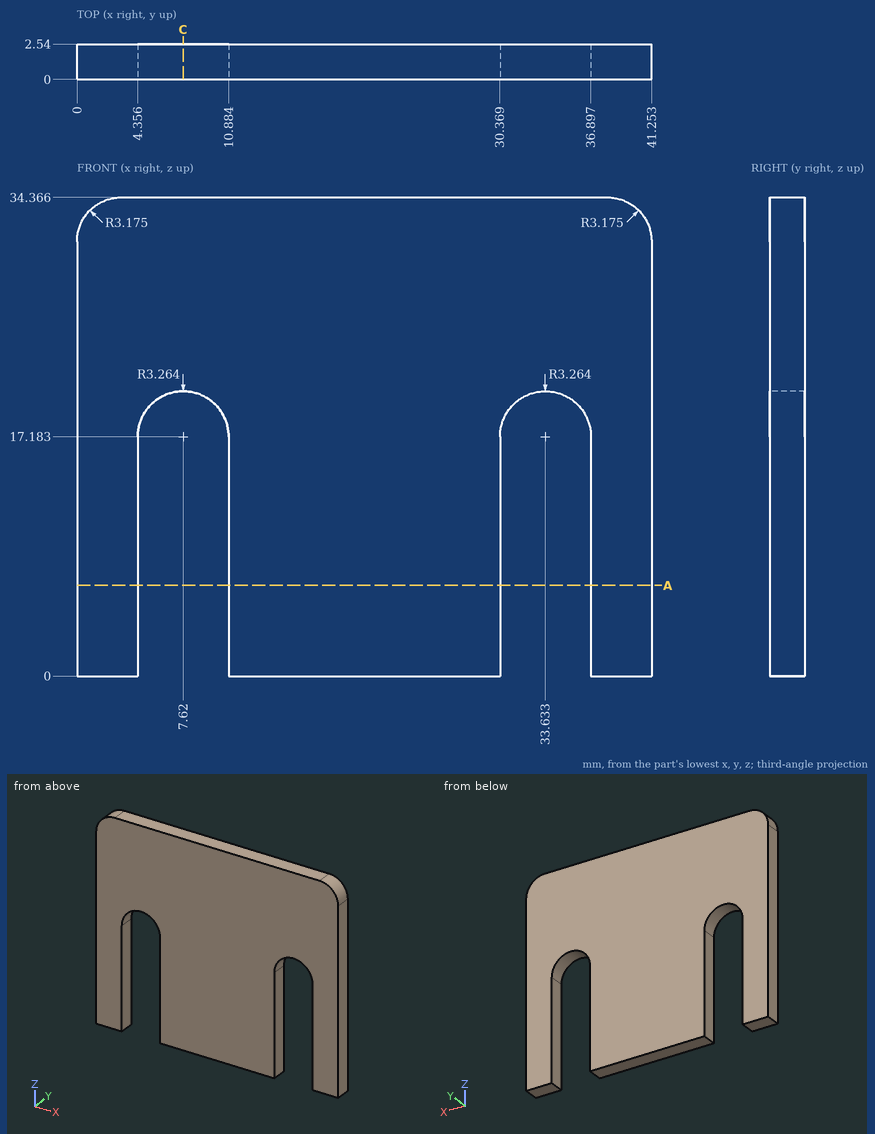
Part print with two shaded views. Sizes in mm from the minimum x, y, z corner. Round coordinates to 2 decimals unless told otherwise and drop trailing zeros. Order: outer loops, then holes, each group sorted by start corner. A loop starts at its lowest first (then second) coordinate and runs counter-clockwise, first axis right, second up. Notation, with made-up numbers: (4.5, 1) - (55.5, 1) arc R17 cw to (55.5, 10) - close; hole circle Ø10 at (-16, 49). An arc over 180 degrees is marked (long way). Return JSON: item names as keys, results as strings.
(1) Cut at A-A (z = 6.5). Give the cut face in (x, y).
Answer key:
{"outline": "(0, 0) - (4.36, 0) - (4.36, 2.54) - (0, 2.54) - close; (10.88, 0) - (30.37, 0) - (30.37, 2.54) - (10.88, 2.54) - close; (36.9, 0) - (41.25, 0) - (41.25, 2.54) - (36.9, 2.54) - close"}
(2) Wall check: probe 1 along X at (y, z) = (1.2, 10); probe 2 along Z at (x, y) = (3, 0.4); probe 3 along X at (y, z) = (2.3, 18). Give the ranges that are in metal, low to high. Write a range as from..to.
Answer key:
{"probe 1": "x = 0..4.36, 10.88..30.37, 36.9..41.25", "probe 2": "z = 0..34.36", "probe 3": "x = 0..4.46, 10.78..30.47, 36.79..41.25"}
(3) Cut at C-C (x = 7.62). Give the cut face in (y, z).
Answer key:
{"outline": "(0, 20.45) - (2.54, 20.45) - (2.54, 34.37) - (0, 34.37) - close"}
(4) Pin check, flat tip, straight feed: pin 1 Ø0.8 at (y, z) = (1, 12.5) entering from -X. Stop position of the tip, or through.
Answer key:
{"pin 1": "stops at x = 0"}
